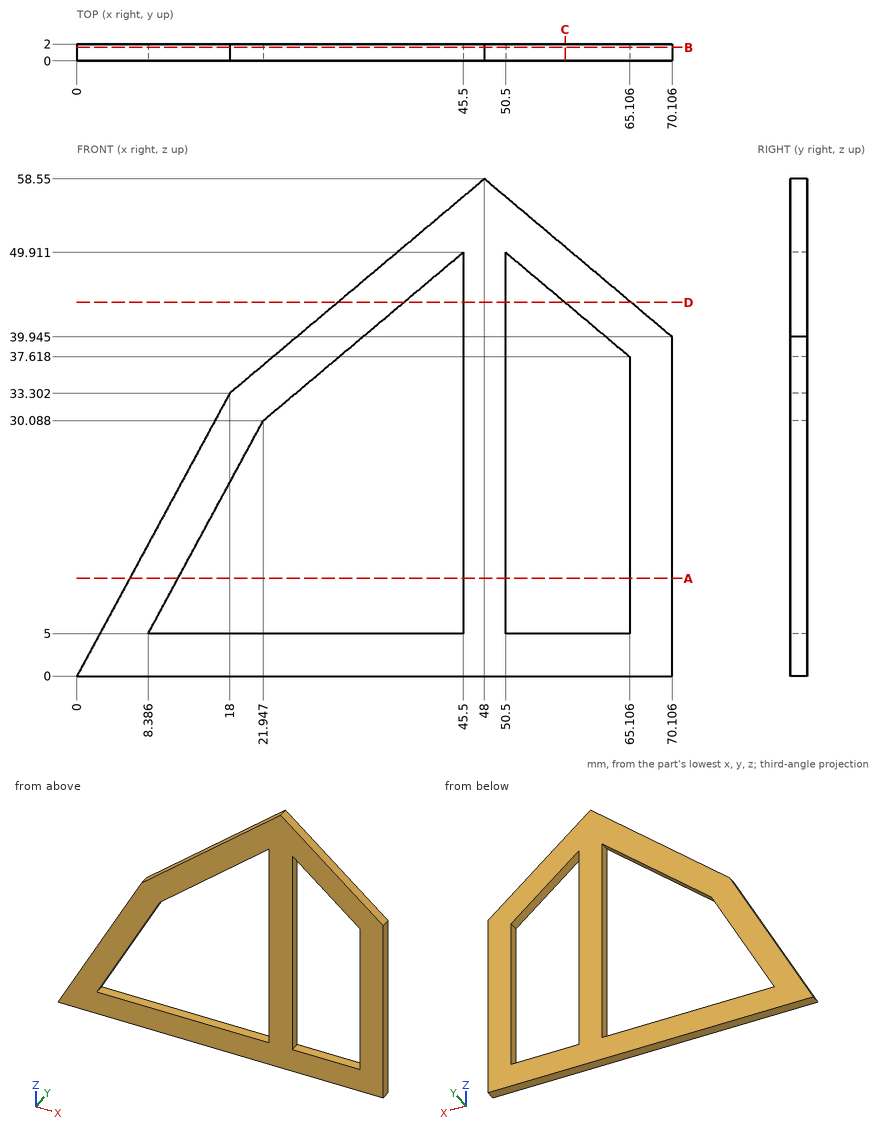
Could you check a few things on this drawing? It's one solid part, dimensions in mm from its lowest x, y, z. Give positions to 0.01 mm unless a question says otherwise; leave off trailing zeros. Order: outer loops, then holes, each group sorted by start corner. A loop starts at its lowest first (then second) coordinate and runs counter-clockwise, first axis right, second up. Notation, with made-up numbers: (22, 76.5) -> (46, 76.5) arc R15 ccw to (46, 99.5) -> close; hole circle Ø9 at (42.5, 44.25). An arc over 180 degrees is marked (long way). Answer in a Markdown table with one row per item. Add a question column.
Item 1: I'm going to push flat-ended pins straight in: P1, Ø1, axis at x = 39.5, y = 0.5, coming from the +Z side; P2, Ø0.6, axis at x = 60, y = 1, coming from the +Z side; P3, Ø0.6, axis at x = 25.5, y = 0.5, coming from the +Z side (1 decimal). Where does each tip first touch, or does it pass through?
Item 2: Imagine slicing it at C-C (x = 57.5). List the corners of the cut face in (y, z) for me (1 decimal).
Item 3: Imagine slicing it at D-D (z = 44). List the corners of the cut face in (x, y) for me.
Item 4: Imagine slicing it at A-A (z = 11.5). List the corners of the cut face in (x, y) for me.
Item 5: Imagine slicing it at B-B (y = 1.6). Count the separate pieces of the cut face and the enclosed holes in it, and give its area (3 significant figures).
Item 6: Please list where these lines run through material, in increasing order: probe 1 along X at (y, z) = (1.75, 41.5) (1 decimal); probe 2 along X at (y, z) = (0.5, 26.5) (1 decimal); probe 3 along Z at (x, y) = (59.5, 1.35) (1 decimal).
Result:
| question | item | result |
|---|---|---|
| 1 | P1 | z = 51.82 |
| 1 | P2 | z = 48.7 |
| 1 | P3 | z = 39.9 |
| 2 | outline | (0, 0) -> (2, 0) -> (2, 5) -> (0, 5) -> close; (0, 44) -> (2, 44) -> (2, 50.6) -> (0, 50.6) -> close |
| 3 | outline | (30.71, 0) -> (38.48, 0) -> (38.48, 2) -> (30.71, 2) -> close; (45.5, 0) -> (50.5, 0) -> (50.5, 2) -> (45.5, 2) -> close; (57.52, 0) -> (65.29, 0) -> (65.29, 2) -> (57.52, 2) -> close |
| 4 | outline | (6.22, 0) -> (11.9, 0) -> (11.9, 2) -> (6.22, 2) -> close; (45.5, 0) -> (50.5, 0) -> (50.5, 2) -> (45.5, 2) -> close; (65.11, 0) -> (70.11, 0) -> (70.11, 2) -> (65.11, 2) -> close |
| 5 | separate pieces | 1 |
| 5 | enclosed holes | 2 |
| 5 | area | 1,210 mm2 |
| 6 | probe 1 | 27.7 to 35.5, 45.5 to 50.5, 60.5 to 68.3 |
| 6 | probe 2 | 14.3 to 20, 45.5 to 50.5, 65.1 to 70.1 |
| 6 | probe 3 | 0 to 5, 42.3 to 48.9 |
